Design review of the part shown in the three views and the two pictorial views. Dimensions are in mm from the part's minimum x, y and z. A direction names the side the tool comes from. Coordinates: 2 decimals unless noted, no trailing zeros. Write each loop counter-clockwise with the first axis right and the second up, starting at its lowest first coordinate (ties: lowest second). Pieces come first, ordered by that corner, then holes. Notation, with made-up numbers: (-33, -28.5) -> (26, -28.5) arc R12 ccw to (26, -16.5) -> close; hole circle Ø8 at (40.5, 12.5). An arc over 180 degrees is marked (long way). Write item = value, one per line. Start each with the question number.
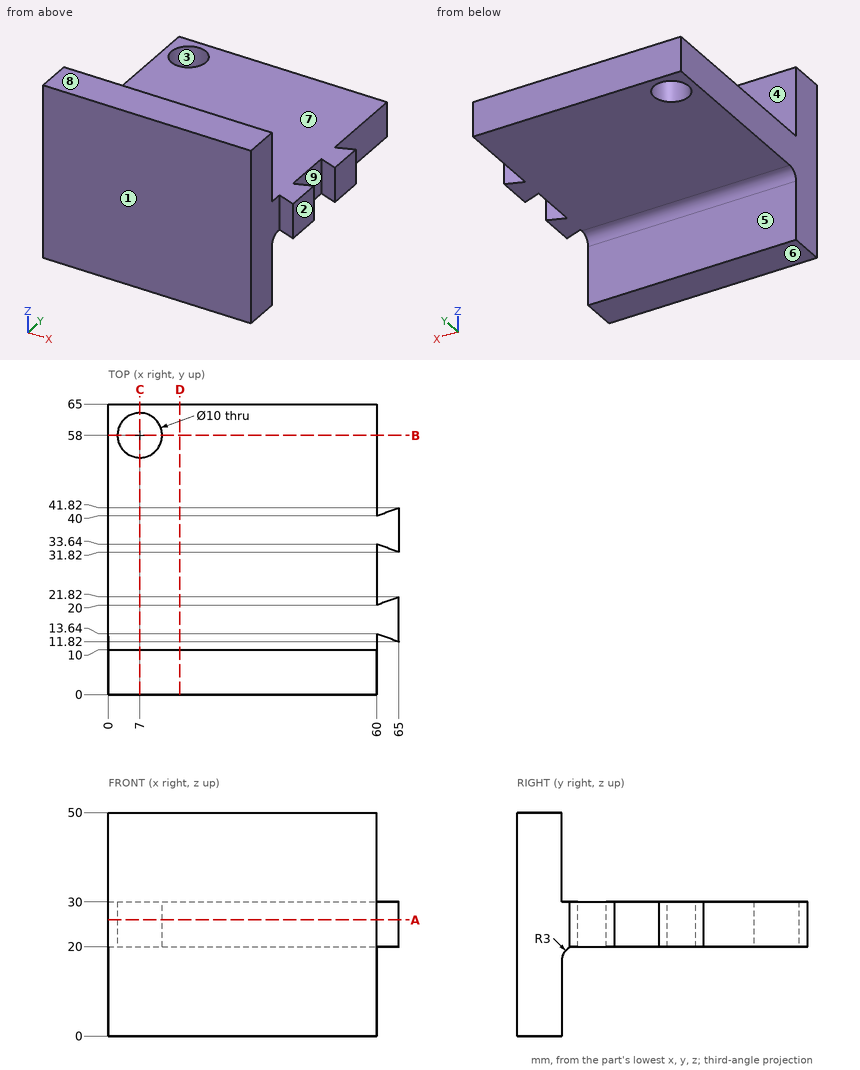
(1) Take a section at B-B, the plane y = 58. State the section outline as (x, z) points, then the cut area to 3 significant figures.
(2) Take a section at D-D, the plane x = 16. State the section outline as (y, z) points.
(3) For pin 1 Ø5 at (x, z) = (51.5, 15) entering from +Y; pin 2 Ø10 at (x, y) = (18, 20.5) entering from +Z; pin 3 Ø16 at (x, y) = (32.5, 34) entering from -Z, all flat-tipped, find the tip position at first contact; note any pin that passes through.
(4) Take a section at A-A, the plane z = 26. State the section outline as (x, y) points, then the cut area to 3 significant figures.
(5) Mouldability with a two-part tool opening along Y and no side actions: class the marked faces 1, 2, 3 and 4 as pulls with the +Y half, pulls with the -Y half, needs draft (parallel to the pull), parting line crosses it, or undercut.
(6) Take a section at C-C, the plane x = 7. State the section outline as (y, z) points.
(7) For the marked faces 5, 6, 7, 8 and 9, list the 3-axis set-ups (+Z, -Z, +X, -X, +Y, -Y) from which the entire face can be reached by the end or side of a thin tool; tool diameter is ignored.
(8) For line 1 (Y direction, x = 7, z = 24); line 2 (Y direction, x = 16, z = 37); line 3 (Z direction, x = 26, y = 23.5), list the stretches that pass through material, from the lowest coordinate up.
Report:
q1.outline = (0, 20) -> (2, 20) -> (2, 30) -> (0, 30) -> close; (12, 20) -> (60, 20) -> (60, 30) -> (12, 30) -> close
q1.area = 500 mm2
q2.outline = (0, 0) -> (10, 0) -> (10, 17) arc R3 cw to (13, 20) -> (65, 20) -> (65, 30) -> (10, 30) -> (10, 50) -> (0, 50) -> close
q3.pin_1 = 10.04
q3.pin_2 = 30
q3.pin_3 = 20
q4.outline = (0, 0) -> (60, 0) -> (60, 13.64) -> (65, 11.82) -> (65, 21.82) -> (60, 20) -> (60, 33.64) -> (65, 31.82) -> (65, 41.82) -> (60, 40) -> (60, 65) -> (0, 65) -> close; hole circle Ø10 at (7, 58)
q4.area = 3,900 mm2
q5.face_1 = pulls with the -Y half
q5.face_2 = needs draft
q5.face_3 = undercut
q5.face_4 = pulls with the +Y half
q6.outline = (0, 0) -> (10, 0) -> (10, 17) arc R3 cw to (13, 20) -> (53, 20) -> (53, 30) -> (10, 30) -> (10, 50) -> (0, 50) -> close; (63, 20) -> (65, 20) -> (65, 30) -> (63, 30) -> close
q7.face_5 = -Z, +X, -X, +Y
q7.face_6 = -Z, +X, -X, +Y, -Y
q7.face_7 = +Z, +X, -X, +Y
q7.face_8 = +Z, +X, -X, +Y, -Y
q7.face_9 = +Z, -Z
q8.line_1 = 0 to 53, 63 to 65
q8.line_2 = 0 to 10
q8.line_3 = 20 to 30
